The model under review builds one solid part; all positions refer to its coordinate system, in mm. Face numbers are marked on the shaded views. A direction names the side the tool comes from. Give positions to 0.01 mm unless a question says otherwise; leave off trailing zeros. Order: outer loops, then holes, each group sorted by start corner. A loop starts at its lowest first (then second) coordinate and runs counter-clockwise, first axis right, second up. Notation, with made-up numbers: (73, 14) - (85, 14) arc R15 cw to (85, 19) - close; hole circle Ø1 at (-3.75, 9.25). An arc over 180 degrees is marked (long way). Use CSV: the item, a comma, the result in double quotes. Start each with the question number.
1. Take a section at A-A, the plane y = 3. State the section outline as (x, z) points.
2. For pin 1 (6 mm diameter, centred on x = 7, z = 4, fed in from +Y); pin 2 (3 mm diameter, centred on x = 4.5, y = -25, fed in from -Z); pin 3 (5.5 mm diameter, centred on x = 12.5, z = 5, fed in from +Y); pin 4 (1.5 mm diameter, centred on y = -24.5, z = 4, fed in from +X), all flat-tipped, find the tip position at first contact; note any pin that passes through.
3. Take a section at B-B, the plane y = 19. State the section outline as (x, z) points.
4. To check wall thickness, follow line 1 (Y direction, x = -8, z = 3); line 2 (Y direction, x = 16.5, z = 3.5); line 3 (Y direction, x = 3.5, z = 6.75). State the ranges of each line that lie inside material, in increasing order. Write a range as [from, to].
5. Machinability: for the marked faces 1, 2, 3, 4 and 5, which of the approach directions +Z, -Z, +X, -X, +Y, -Y give a long, thin tool a straight path to every point of the face, cutting with its end or side? Answer none if there is none.
6. Draft analysis for pull direction Y (two halves, no side actions). For the marked faces 6 and 7, state which applies: released by +Y, released by -Y, zero draft, split by the parting line, or undercut.
7. Take a section at D-D, the plane z = 9. State the section outline as (x, y) points, then the cut area to 3 significant figures.
8. Take a section at C-C, the plane x = 15. State the section outline as (y, z) points, then the cut area to 3 significant figures.
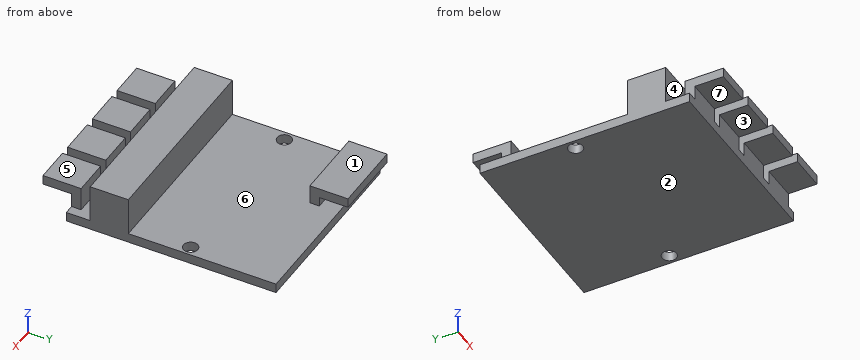
```python
from build123d import *

# Parameters (mm, degrees)
ESQUISSE1_W             = 40
ESQUISSE1_H             = 44
BOSS_EXTRU_1_DEPTH      = 2
ESQUISSE2_W             = 40
ESQUISSE2_H             = 8
BOSS_EXTRU_2_DEPTH      = 8
ESQUISSE3_W             = 36
ESQUISSE3_H             = 2
BOSS_EXTRU_3_DEPTH      = 5
ESQUISSE4_W             = 36
ESQUISSE4_H             = 2
BOSS_EXTRU_4_DEPTH      = 6
ENL_V_MAT_EXTRU_1_REACH = 56.772
ESQUISSE5_W             = 2
ESQUISSE5_H             = 5
ESQUISSE6_W             = 15
ESQUISSE6_H             = 2
BOSS_EXTRU_5_DEPTH      = 4
ESQUISSE7_W             = 15
ESQUISSE7_H             = 2
BOSS_EXTRU_6_DEPTH      = 6
ENL_V_MAT_EXTRU_2_REACH = 37.327
ESQUISSE8_R             = 1.5


with BuildPart() as part:
    # Esquisse1 → Boss.-Extru.1 (new body)
    with BuildSketch(Plane.XY):
        Rectangle(ESQUISSE1_W, ESQUISSE1_H)
    extrude(amount=BOSS_EXTRU_1_DEPTH)

    # Esquisse2 → Boss.-Extru.2 (add)
    with BuildSketch(Plane.XY.offset(2)):
        with Locations((0, -13)):
            Rectangle(ESQUISSE2_W, ESQUISSE2_H)
    extrude(amount=BOSS_EXTRU_2_DEPTH)

    # Esquisse3 → Boss.-Extru.3 (add)
    with BuildSketch(Plane.XY.offset(2)):
        with Locations((0, -21)):
            Rectangle(ESQUISSE3_W, ESQUISSE3_H)
    extrude(amount=BOSS_EXTRU_3_DEPTH)

    # Esquisse4 → Boss.-Extru.4 (add)
    with BuildSketch(Plane.XZ.offset(22)):
        with Locations((0, 6)):
            Rectangle(ESQUISSE4_W, ESQUISSE4_H)
    extrude(amount=BOSS_EXTRU_4_DEPTH)

    # Esquisse5 → Enlèv. mat.-Extru.1 (cut, up to next)
    with BuildSketch(Plane.XZ.offset(28), mode=Mode.PRIVATE) as enl_v_mat_extru_1_sk1:
        with Locations((-9.5, 4.5)):
            Rectangle(ESQUISSE5_W, ESQUISSE5_H)
    enl_v_mat_extru_1_tool1 = extrude(enl_v_mat_extru_1_sk1.sketch, amount=-ENL_V_MAT_EXTRU_1_REACH, mode=Mode.PRIVATE) & part.part
    # Esquisse5 → Enlèv. mat.-Extru.1 (cut, up to next)
    with BuildSketch(Plane.XZ.offset(28), mode=Mode.PRIVATE) as enl_v_mat_extru_1_sk2:
        with Locations((0, 4.5)):
            Rectangle(ESQUISSE5_W, ESQUISSE5_H)
    enl_v_mat_extru_1_tool2 = extrude(enl_v_mat_extru_1_sk2.sketch, amount=-ENL_V_MAT_EXTRU_1_REACH, mode=Mode.PRIVATE) & part.part
    # Esquisse5 → Enlèv. mat.-Extru.1 (cut, up to next)
    with BuildSketch(Plane.XZ.offset(28), mode=Mode.PRIVATE) as enl_v_mat_extru_1_sk3:
        with Locations((9.5, 4.5)):
            Rectangle(ESQUISSE5_W, ESQUISSE5_H)
    enl_v_mat_extru_1_tool3 = extrude(enl_v_mat_extru_1_sk3.sketch, amount=-ENL_V_MAT_EXTRU_1_REACH, mode=Mode.PRIVATE) & part.part
    add(enl_v_mat_extru_1_tool1.solids().sort_by_distance((-9.5, -28, 4.5))[0], mode=Mode.SUBTRACT)
    add(enl_v_mat_extru_1_tool2.solids().sort_by_distance((0, -28, 4.5))[0], mode=Mode.SUBTRACT)
    add(enl_v_mat_extru_1_tool3.solids().sort_by_distance((9.5, -28, 4.5))[0], mode=Mode.SUBTRACT)

    # Esquisse6 → Boss.-Extru.5 (add)
    with BuildSketch(Plane.XY.offset(2)):
        with Locations((-11.5, 17)):
            Rectangle(ESQUISSE6_W, ESQUISSE6_H)
    extrude(amount=BOSS_EXTRU_5_DEPTH)

    # Esquisse7 → Boss.-Extru.6 (add)
    with BuildSketch(Plane(origin=(0, 18, 0), x_dir=(1, 0, 0), z_dir=(0, 1, 0))):
        with Locations((-11.5, -5)):
            Rectangle(ESQUISSE7_W, ESQUISSE7_H)
    extrude(amount=BOSS_EXTRU_6_DEPTH)

    # Esquisse8 → Enlèv. mat.-Extru.2 (cut, up to next)
    with BuildSketch(Plane.XY.offset(2), mode=Mode.PRIVATE) as enl_v_mat_extru_2_sk1:
        with Locations((18, 3)):
            Circle(ESQUISSE8_R)
    enl_v_mat_extru_2_tool1 = extrude(enl_v_mat_extru_2_sk1.sketch, amount=-ENL_V_MAT_EXTRU_2_REACH, mode=Mode.PRIVATE) & part.part
    enl_v_mat_extru_2 = enl_v_mat_extru_2_tool1.solids().sort_by_distance((18, 3, 2))[0]
    add(enl_v_mat_extru_2, mode=Mode.SUBTRACT)

    # Symétrie1: Enlèv. mat.-Extru.2 across plane
    add(enl_v_mat_extru_2.mirror(Plane(origin=(0, 0, 0), x_dir=(0, 0, 1), z_dir=(1, 0, 0))), mode=Mode.SUBTRACT)


solid = part.part
```
Determined:
1,outline,"(-20, 0) - (-19.5, 0) - (-19.5, 2) - (-20, 2) - close; (-16.5, 0) - (16.5, 0) - (16.5, 2) - (-16.5, 2) - close; (19.5, 0) - (20, 0) - (20, 2) - (19.5, 2) - close"
2,pin 1,"stops at y = 22"
2,pin 2,"stops at z = 5"
2,pin 3,"stops at y = -9"
2,pin 4,"passes through"
3,outline,"(-20, 0) - (20, 0) - (20, 2) - (-20, 2) - close; (-19, 4) - (-4, 4) - (-4, 6) - (-19, 6) - close"
4,line 1,"y = [-22, -20], [-17, -9], [16, 18]"
4,line 2,"y = [-22, -20], [-17, -9]"
4,line 3,"y = [-28, -20], [-17, -9]"
5,face 1,"+Z, +X, -X, +Y"
5,face 2,"-Z, +X, -X, +Y, -Y"
5,face 3,"-Z, +X, -X, -Y"
5,face 4,"+Z, +X, -X"
5,face 5,"+Z, +X, -X, -Y"
6,face 6,"undercut"
6,face 7,"zero draft"
7,outline,"(-20, -17) - (20, -17) - (20, -9) - (-20, -9) - close"
7,area,"320 mm²"
8,outline,"(-28, 5) - (-22, 5) - (-22, 0) - (22, 0) - (22, 2) - (-9, 2) - (-9, 10) - (-17, 10) - (-17, 2) - (-20, 2) - (-20, 7) - (-28, 7) - close"
8,area,"174 mm²"
